Could you check a few things on this drawing? It's one solid part, dimensions in mm from its lowest x, y, z. Give positions to 0.01 mm unless a question says otherwise; leave off trailing zeros. Loops run counter-clockwise (first coordinate to the right, second up) from the corner with the lowest first, then second, coordinate; pieces in that order, holes last.
1. Imagine slicing it at B-B (z = 2.25). List the corners of the cut face in (x, y) for me.
2. Imagine slicing it at C-C (x = 3). List the corners of the cut face in (y, z) for me, plus the area to 3 significant figures.
3. For P1, Ø1, axis at x = 7.5, y = 7, coming from the -Z side; P2, Ø2.5, axis at x = 15, y = 4, coming from the -Z side, each with a flat end and sliding along its axis, tell me the tip position at first contact or that it passes through.
4. I need wall thicknesses on line 1 along Y through (x, z) = (15, 2.4); line 2 along X through (y, z) = (3.25, 1.7); line 3 along X through (y, z) = (5.25, 1). Which ranges of each line are inside material? Lowest first, please.
5. Imagine slicing it at A-A (y = 4). List the corners of the cut face in (x, z) for me, plus the area to 3 significant figures.
6. Thinking about a two-plate mould opening in Y: for the marked faces 1, 2, 3 and 4, which applies, +Y half, -Y half, draft (parallel to the pull), parting line (faces both ways), or undercut?
7. Imagine slicing it at D-D (y = 2.75). List the corners of the cut face in (x, z) for me, plus the area to 3 significant figures.
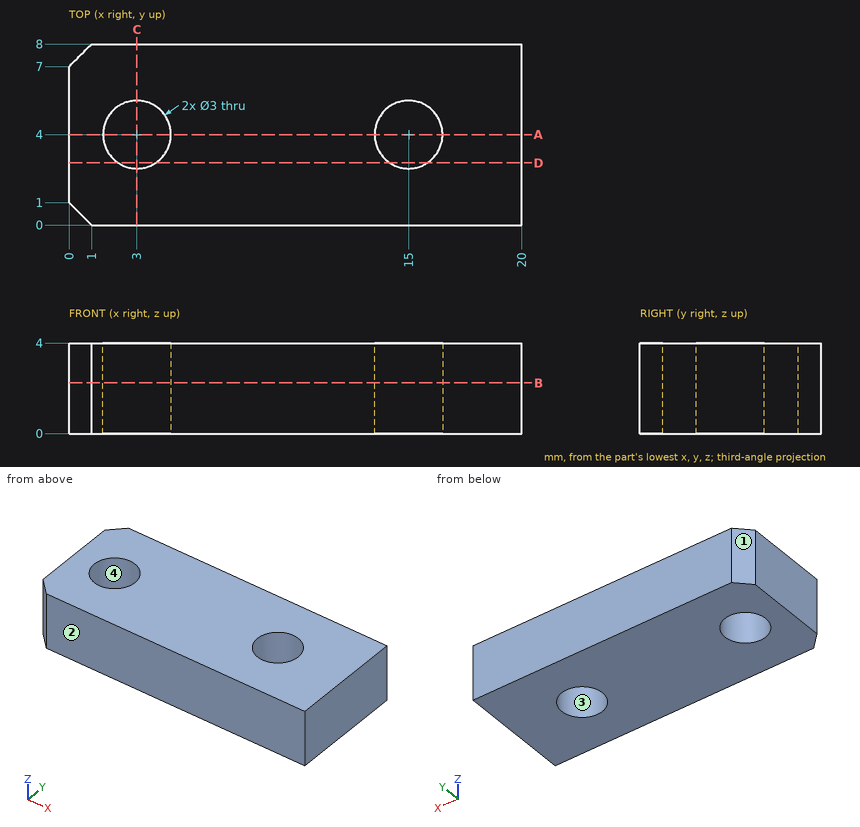
Derived:
1. outline: (0, 1) - (1, 0) - (20, 0) - (20, 8) - (1, 8) - (0, 7) - close; hole circle Ø3 at (3, 4); hole circle Ø3 at (15, 4)
2. outline: (0, 0) - (2.5, 0) - (2.5, 4) - (0, 4) - close; (5.5, 0) - (8, 0) - (8, 4) - (5.5, 4) - close
2. area: 20.0 mm2
3. P1: stops at z = 0
3. P2: passes through
4. line 1: y = 0 to 2.5, 5.5 to 8
4. line 2: x = 0 to 1.7, 4.3 to 13.7, 16.3 to 20
4. line 3: x = 0 to 2.17, 3.83 to 14.17, 15.83 to 20
5. outline: (0, 0) - (1.5, 0) - (1.5, 4) - (0, 4) - close; (4.5, 0) - (13.5, 0) - (13.5, 4) - (4.5, 4) - close; (16.5, 0) - (20, 0) - (20, 4) - (16.5, 4) - close
5. area: 56.0 mm2
6. face 1: +Y half
6. face 2: -Y half
6. face 3: undercut
6. face 4: undercut
7. outline: (0, 0) - (2.17, 0) - (2.17, 4) - (0, 4) - close; (3.83, 0) - (14.17, 0) - (14.17, 4) - (3.83, 4) - close; (15.83, 0) - (20, 0) - (20, 4) - (15.83, 4) - close
7. area: 66.7 mm2
